```python
from build123d import *

# Parameters (mm, degrees)
SKIZZE1_W                                  = 130
SKIZZE1_H                                  = 80
AUFSATZ_LINEAR_AUSTRAGEN1_DEPTH            = 60
SKIZZE2_W                                  = 118
SKIZZE2_H                                  = 66.841692054
SCHNITT_LINEAR_AUSTRAGEN1_DEPTH            = 55
SKIZZE3_W                                  = 15.6
SKIZZE3_H                                  = 20
AUFSATZ_LINEAR_AUSTRAGEN2_DEPTH            = 6.8
SCHNITT_LINEAR_START                       = -20
SCHNITT_LINEAR_AUSTRAGEN10_DEPTH           = 20
SCHNITT_LINEAR_AUSTRAGEN11_DEPTH           = 20
SKIZZE16_W                                 = 15.6
SKIZZE16_H                                 = 20
AUFSATZ_LINEAR_AUSTRAGEN3_DEPTH            = 6.8
SCHNITT_LINEAR_AUSTRAGEN12_DEPTH           = 20
SCHNITT_LINEAR_AUSTRAGEN13_DEPTH           = 20
SKIZZE21_W                                 = 30
SKIZZE21_H                                 = 20
SCHNITT_LINEAR_AUSTRAGEN14_DEPTH           = 10
SKIZZE23_W                                 = 3
SKIZZE23_H                                 = 6
SCHNITT_LINEAR_AUSTRAGEN16_DEPTH           = 8
SKIZZE24_W                                 = 3
SKIZZE24_H                                 = 6
SCHNITT_LINEAR_AUSTRAGEN17_DEPTH           = 8
F_3_4_3_4_DURCHMESSER_BOHRUNG2_D           = 3.4
F_3_4_3_4_DURCHMESSER_BOHRUNG2_DEPTH       = 10
F_3_4_3_4_DURCHMESSER_BOHRUNG2_CSINK_D     = 3.45
F_3_4_3_4_DURCHMESSER_BOHRUNG2_CSINK_ANGLE = 90
F_3_4_3_4_DURCHMESSER_BOHRUNG2_TIP         = 1.021463052
F_2_4_2_4_DURCHMESSER_BOHRUNG1_D           = 2.4
F_2_4_2_4_DURCHMESSER_BOHRUNG1_DEPTH       = 10
F_2_4_2_4_DURCHMESSER_BOHRUNG1_CSINK_D     = 2.45
F_2_4_2_4_DURCHMESSER_BOHRUNG1_CSINK_ANGLE = 90
F_2_4_2_4_DURCHMESSER_BOHRUNG1_TIP         = 0.721032743
SKIZZE33_W                                 = 5
SKIZZE33_H                                 = 2
SCHNITT_LINEAR_AUSTRAGEN18_DEPTH           = 5.5
SKIZZE22_W                                 = 30
SKIZZE22_H                                 = 20
SCHNITT_LINEAR_AUSTRAGEN19_DEPTH           = 34.5
F_3_4_3_4_DURCHMESSER_BOHRUNG3_D           = 3.4
F_3_4_3_4_DURCHMESSER_BOHRUNG3_DEPTH       = 10
F_3_4_3_4_DURCHMESSER_BOHRUNG3_CSINK_D     = 3.45
F_3_4_3_4_DURCHMESSER_BOHRUNG3_CSINK_ANGLE = 90
F_3_4_3_4_DURCHMESSER_BOHRUNG3_TIP         = 1.021463052
SKIZZE37_W                                 = 5
SKIZZE37_H                                 = 2
SCHNITT_LINEAR_AUSTRAGEN21_DEPTH           = 5.5
SKIZZE38_W                                 = 5
SKIZZE38_H                                 = 2
SCHNITT_LINEAR_AUSTRAGEN22_DEPTH           = 5.5
SKIZZE39_W                                 = 5
SKIZZE39_H                                 = 2
SCHNITT_LINEAR_AUSTRAGEN23_DEPTH           = 5.5
VERRUNDUNG3_R                              = 3


# Read off the part's stored shape, not the designer's step: Schnitt-Linear austragen10, Schnitt-Linear austragen11, Schnitt-Linear austragen12, Schnitt-Linear austragen13
with BuildPart() as part:
    # Skizze1 → Aufsatz-Linear austragen1 (new body)
    with BuildSketch(Plane(origin=(0, 0, 0), x_dir=(1, 0, 0), z_dir=(0, 1, 0))):
        with Locations((65, 38.841692054)):
            Rectangle(SKIZZE1_W, SKIZZE1_H)
    extrude(amount=AUFSATZ_LINEAR_AUSTRAGEN1_DEPTH)

    # Skizze2 → Schnitt-Linear austragen1 (cut)
    with BuildSketch(Plane(origin=(0, 60, 0), x_dir=(1, 0, 0), z_dir=(0, 1, 0))):
        with Locations((65, 39.420846027)):
            Rectangle(SKIZZE2_W, SKIZZE2_H)
    extrude(amount=-SCHNITT_LINEAR_AUSTRAGEN1_DEPTH, mode=Mode.SUBTRACT)

    # Skizze3 → Aufsatz-Linear austragen2 (add)
    with BuildSketch(Plane(origin=(0, 5, 0), x_dir=(1, 0, 0), z_dir=(0, 1, 0))):
        with Locations((57.2, 38.841692054)):
            Rectangle(SKIZZE3_W, SKIZZE3_H)
    extrude(amount=AUFSATZ_LINEAR_AUSTRAGEN2_DEPTH)

    # Schnitt-Linear austragen10 outline → Schnitt-Linear austragen10 (cut)
    with BuildSketch(Plane.XY.offset(-28.841692054).offset(SCHNITT_LINEAR_START)):
        Polygon((49.4, 5), (53.32598183, 11.8), (49.4, 11.8), align=None)
    extrude(amount=SCHNITT_LINEAR_AUSTRAGEN10_DEPTH, mode=Mode.SUBTRACT)

    # Schnitt-Linear austragen11 outline → Schnitt-Linear austragen11 (cut)
    with BuildSketch(Plane.XY.offset(-28.841692054).offset(SCHNITT_LINEAR_START)):
        Polygon((53.32598183, 11.8), (65, 5), (65, 11.8), align=None)
    extrude(amount=SCHNITT_LINEAR_AUSTRAGEN11_DEPTH, mode=Mode.SUBTRACT)

    # Skizze16 → Aufsatz-Linear austragen3 (add)
    with BuildSketch(Plane(origin=(0, 5, 0), x_dir=(1, 0, 0), z_dir=(0, 1, 0))):
        with Locations((72.8, 38.841692054)):
            Rectangle(SKIZZE16_W, SKIZZE16_H)
    extrude(amount=AUFSATZ_LINEAR_AUSTRAGEN3_DEPTH)

    # Schnitt-Linear austragen12 outline → Schnitt-Linear austragen12 (cut)
    with BuildSketch(Plane.XY.offset(-28.841692054).offset(SCHNITT_LINEAR_START)):
        Polygon((80.6, 11.8), (76.67401817, 11.8), (80.6, 5), align=None)
    extrude(amount=SCHNITT_LINEAR_AUSTRAGEN12_DEPTH, mode=Mode.SUBTRACT)

    # Schnitt-Linear austragen13 outline → Schnitt-Linear austragen13 (cut)
    with BuildSketch(Plane.XY.offset(-28.841692054).offset(SCHNITT_LINEAR_START)):
        Polygon((65, 5), (76.67401817, 11.8), (65, 11.8), align=None)
    extrude(amount=SCHNITT_LINEAR_AUSTRAGEN13_DEPTH, mode=Mode.SUBTRACT)

    # Skizze21 → Schnitt-Linear austragen14 (cut)
    with BuildSketch(Plane(origin=(0, 5, 0), x_dir=(1, 0, 0), z_dir=(0, 1, 0))):
        with Locations((95.6, 38.841692054)):
            Rectangle(SKIZZE21_W, SKIZZE21_H)
    extrude(amount=-SCHNITT_LINEAR_AUSTRAGEN14_DEPTH, mode=Mode.SUBTRACT)

    # Skizze23 → Schnitt-Linear austragen16 (cut)
    with BuildSketch(Plane(origin=(14.292377765, -24.536687899, 0), x_dir=(0.8640958560374116, 0.5033272807815734, 0), z_dir=(-0.5033272807815734, 0.8640958560374116, 0))):
        with Locations((66.882744729, 38.841692054)):
            Rectangle(SKIZZE23_W, SKIZZE23_H)
    extrude(amount=-SCHNITT_LINEAR_AUSTRAGEN16_DEPTH, mode=Mode.SUBTRACT)

    # Skizze24 → Schnitt-Linear austragen17 (cut)
    with BuildSketch(Plane(origin=(18.64160794, 32.003304383, 0), x_dir=(0.8640958560374131, -0.5033272807815709, 0), z_dir=(0.5033272807815709, 0.8640958560374132, 0))):
        with Locations((45.934845453, 38.841692054)):
            Rectangle(SKIZZE24_W, SKIZZE24_H)
    extrude(amount=-SCHNITT_LINEAR_AUSTRAGEN17_DEPTH, mode=Mode.SUBTRACT)

    # Ø3.4 (3.4) Durchmesser Bohrung2
    with Locations(Plane(origin=(62.615063509, 36.150823773, 0), x_dir=(0, 0, -1), z_dir=(0.8660254037844358, 0.5000000000000049, 0))):
        with Locations((38.841692054, -32.069872981)):
            CounterSinkHole(F_3_4_3_4_DURCHMESSER_BOHRUNG2_D / 2, F_3_4_3_4_DURCHMESSER_BOHRUNG2_CSINK_D / 2, depth=F_3_4_3_4_DURCHMESSER_BOHRUNG2_DEPTH, counter_sink_angle=F_3_4_3_4_DURCHMESSER_BOHRUNG2_CSINK_ANGLE)
            with Locations((0, 0, -(F_3_4_3_4_DURCHMESSER_BOHRUNG2_DEPTH + F_3_4_3_4_DURCHMESSER_BOHRUNG2_TIP / 2))):  # 118° drill point
                Cone(0, F_3_4_3_4_DURCHMESSER_BOHRUNG2_D / 2, F_3_4_3_4_DURCHMESSER_BOHRUNG2_TIP, mode=Mode.SUBTRACT)

    # Ø2.4 (2.4) Durchmesser Bohrung1
    with Locations(Plane(origin=(0, 60, 0), x_dir=(1, 0, 0), z_dir=(0, 1, 0))):
        with Locations((127, 38.841692054), (95, 75.841692054), (35, 75.841692054), (35, 3), (95, 3), (3, 38.841692054), (132.023901178, -13.702298919)):
            CounterSinkHole(F_2_4_2_4_DURCHMESSER_BOHRUNG1_D / 2, F_2_4_2_4_DURCHMESSER_BOHRUNG1_CSINK_D / 2, depth=F_2_4_2_4_DURCHMESSER_BOHRUNG1_DEPTH, counter_sink_angle=F_2_4_2_4_DURCHMESSER_BOHRUNG1_CSINK_ANGLE)
            with Locations((0, 0, -(F_2_4_2_4_DURCHMESSER_BOHRUNG1_DEPTH + F_2_4_2_4_DURCHMESSER_BOHRUNG1_TIP / 2))):  # 118° drill point
                Cone(0, F_2_4_2_4_DURCHMESSER_BOHRUNG1_D / 2, F_2_4_2_4_DURCHMESSER_BOHRUNG1_TIP, mode=Mode.SUBTRACT)

    # Skizze33 → Schnitt-Linear austragen18 (cut)
    with BuildSketch(Plane(origin=(0, 0, -78.841692054), x_dir=(-1, 0, 0), z_dir=(0, 0, -1))):
        with Locations((-95, 56)):
            Rectangle(SKIZZE33_W, SKIZZE33_H)
        with Locations((-35, 56)):
            Rectangle(SKIZZE33_W, SKIZZE33_H)
    extrude(amount=-SCHNITT_LINEAR_AUSTRAGEN18_DEPTH, mode=Mode.SUBTRACT)

    # Skizze22 → Schnitt-Linear austragen19 (cut)
    with BuildSketch(Plane(origin=(0, 5, 0), x_dir=(1, 0, 0), z_dir=(0, 1, 0))):
        with Locations((34.4, 38.841692054)):
            Rectangle(SKIZZE22_W, SKIZZE22_H)
    extrude(amount=-SCHNITT_LINEAR_AUSTRAGEN19_DEPTH, mode=Mode.SUBTRACT)

    # Ø3.4 (3.4) Durchmesser Bohrung3
    with Locations(Plane(origin=(34.884936491, -20.140827473, 0), x_dir=(0, 0, 1), z_dir=(-0.8660254037844404, 0.49999999999999695, 0))):
        with Locations((-38.841692054, 32.930127019)):
            CounterSinkHole(F_3_4_3_4_DURCHMESSER_BOHRUNG3_D / 2, F_3_4_3_4_DURCHMESSER_BOHRUNG3_CSINK_D / 2, depth=F_3_4_3_4_DURCHMESSER_BOHRUNG3_DEPTH, counter_sink_angle=F_3_4_3_4_DURCHMESSER_BOHRUNG3_CSINK_ANGLE)
            with Locations((0, 0, -(F_3_4_3_4_DURCHMESSER_BOHRUNG3_DEPTH + F_3_4_3_4_DURCHMESSER_BOHRUNG3_TIP / 2))):  # 118° drill point
                Cone(0, F_3_4_3_4_DURCHMESSER_BOHRUNG3_D / 2, F_3_4_3_4_DURCHMESSER_BOHRUNG3_TIP, mode=Mode.SUBTRACT)

    # Skizze37 → Schnitt-Linear austragen21 (cut)
    with BuildSketch(Plane.XY.offset(1.158307946)):
        with Locations((35, 56)):
            Rectangle(SKIZZE37_W, SKIZZE37_H)
        with Locations((95, 56)):
            Rectangle(SKIZZE37_W, SKIZZE37_H)
    extrude(amount=-SCHNITT_LINEAR_AUSTRAGEN21_DEPTH, mode=Mode.SUBTRACT)

    # Skizze38 → Schnitt-Linear austragen22 (cut)
    with BuildSketch(Plane(origin=(130, 0, 0), x_dir=(0, 0, -1), z_dir=(1, 0, 0))):
        with Locations((38.841692054, 56)):
            Rectangle(SKIZZE38_W, SKIZZE38_H)
    extrude(amount=-SCHNITT_LINEAR_AUSTRAGEN22_DEPTH, mode=Mode.SUBTRACT)

    # Skizze39 → Schnitt-Linear austragen23 (cut)
    with BuildSketch(Plane.ZY):
        with Locations((-38.841692054, 56)):
            Rectangle(SKIZZE39_W, SKIZZE39_H)
    extrude(amount=-SCHNITT_LINEAR_AUSTRAGEN23_DEPTH, mode=Mode.SUBTRACT)

    # Verrundung3
    verrundung3_edges = [part.edges().sort_by_distance(p)[0] for p in [
        (6, 5, -39.420846027),
        (65, 5, -72.841692054),
        (124, 5, -39.420846027),
        (65, 5, -6),
    ]]
    fillet(verrundung3_edges, radius=VERRUNDUNG3_R)


solid = part.part
```
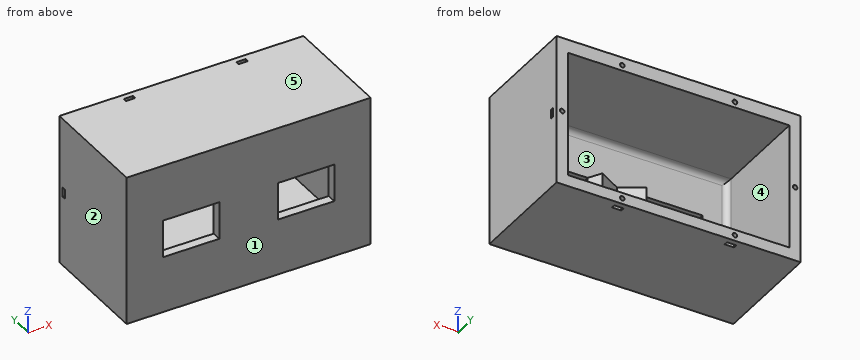
For this review, take the finished solid that the model builds, in its own axes (mm). Face numbers are marked on the shaded views. A direction names the side the tool comes from. Round coordinates to 2 decimals unless told otherwise and drop trailing zeros. Write each loop counter-clockwise with the first axis right and the second up, starting at its lowest first coordinate (ties: lowest second). Pieces come first, ordered by that corner, then holes. Notation, with made-up numbers: (76.5, -0.75) -> (86.5, -0.75) arc R9 ccw to (86.5, 8.25) -> close; hole circle Ø2 at (44.5, -6). An arc over 180 degrees is marked (long way). Use one line per item in the form item = value.
Q1. To check wall thickness, follow probe 1 along Z at (x, y) = (95, 51); probe 2 along Z at (x, y) = (110, 15.5); probe 3 along X at (y, z) = (35.5, -53). State the ranges of each line that lie inside material, in increasing order. Write a range as from..to.
Resolved:
probe_1 = -78.84..-77.04, -74.64..-72.84, -6..-4.2, -1.8..1.16
probe_2 = -78.84..-72.84, -6..1.16
probe_3 = 0..6, 124..130
Q2. Machinability: for the marked faces 4 and 5, which of the approach directions +Z, -Z, +X, -X, +Y, -Y give a long, thin tool a straight path to every point of the face, cutting with its end or side? Answer none if there is none.
Resolved:
face_4 = +Y
face_5 = +Z, +X, -X, +Y, -Y
Q3. Clearance check with a flat-ended pin moving along its axis: pin 1 Ø10 at (x, z) = (77, -55) entering from +Y. State where the tip first meets the part, or that it passes through.
Resolved:
pin_1 = 5
Q4. The part is to be moulded in two halves that separate along X. For the marked faces 1, 2 and 3, say which applies: released by +X, released by -X, zero draft, split by the parting line, or undercut.
Resolved:
face_1 = zero draft
face_2 = released by -X
face_3 = undercut
Q5. Consider section A-A (x = 87). State the section outline as (y, z) points, then the cut area to 3 significant figures.
Resolved:
outline = (0, -78.84) -> (60, -78.84) -> (60, -72.84) -> (8, -72.84) arc R3 cw to (5, -69.84) -> (5, -48.84) -> (0, -48.84) -> close; (0, -28.84) -> (5, -28.84) -> (5, -9) arc R3 cw to (8, -6) -> (60, -6) -> (60, 1.16) -> (0, 1.16) -> close
area = 1,030 mm²
Q6. Consider section B-B (y = 47). State the section outline as (x, z) points.
Resolved:
outline = (0, -78.84) -> (130, -78.84) -> (130, 1.16) -> (0, 1.16) -> close; hole (6, -72.84) -> (124, -72.84) -> (124, -6) -> (6, -6) -> close
Q7. Consider section C-C (z = -56.5). State the section outline as (x, y) points, then the cut area to 3 significant figures.
Resolved:
outline = (0, 0) -> (130, 0) -> (130, 60) -> (124, 60) -> (124, 8) arc R3 cw to (121, 5) -> (9, 5) arc R3 cw to (6, 8) -> (6, 60) -> (0, 60) -> close
area = 1,310 mm²
